```python
from build123d import *

# Parameters (mm, degrees)
SKETCH1_R           = 12.6365
BOSS_EXTRUDE1_DEPTH = 12.7
SKETCH2_R           = 17.4625
BOSS_EXTRUDE2_DEPTH = 12.7
SKETCH3_R           = 11.1125
CUT_EXTRUDE1_DEPTH  = 7.112
SKETCH4_R           = 7.27458794
CUT_EXTRUDE2_DEPTH  = 0.2
SKETCH5_R           = 5.08
CUT_EXTRUDE3_DEPTH  = 31.611330525
CHAMFER1_SIZE       = 0.4


with BuildPart() as part:
    # Sketch1 → Boss-Extrude1 (new body)
    with BuildSketch(Plane(origin=(0, 0, 0), x_dir=(0, 0, -1), z_dir=(1, 0, 0))):
        Circle(SKETCH1_R)
    extrude(amount=BOSS_EXTRUDE1_DEPTH)

    # Sketch2 → Boss-Extrude2 (add)
    with BuildSketch(Plane.ZY):
        Circle(SKETCH2_R)
    extrude(amount=BOSS_EXTRUDE2_DEPTH)

    # Sketch3 → Cut-Extrude1 (cut)
    with BuildSketch(Plane.ZY.offset(12.7)):
        Circle(SKETCH3_R)
    extrude(amount=-CUT_EXTRUDE1_DEPTH, mode=Mode.SUBTRACT)

    # Sketch4 → Cut-Extrude2 (cut)
    with BuildSketch(Plane.ZY.offset(5.588)):
        Circle(SKETCH4_R)
    extrude(amount=-CUT_EXTRUDE2_DEPTH, mode=Mode.SUBTRACT)

    # Sketch5 → Cut-Extrude3 (cut, through all)
    with BuildSketch(Plane.ZY.offset(5.388)):
        Circle(SKETCH5_R)
    extrude(amount=-CUT_EXTRUDE3_DEPTH, mode=Mode.SUBTRACT)

    # Sketch6 → Cut-Revolve1 (revolve, cut)
    with BuildSketch(Plane.XY, mode=Mode.PRIVATE) as cut_revolve1_sk:
        with BuildLine():
            Line((-8.389999984, 17.4625), (-8.389999984, 14.96249992))
            ThreePointArc((-8.389999984, 14.96249992), (-6.35, 12.922499936), (-4.310000016, 14.96249992))
            Line((-4.310000016, 14.96249992), (-4.310000016, 17.4625))
            Line((-4.310000016, 17.4625), (-8.389999984, 17.4625))
        make_face()
    revolve(cut_revolve1_sk.sketch.rotate(Axis((-6.35, 0, 0), (1, 0, 0)), 90), axis=Axis((-6.35, 0, 0), (1, 0, 0)), mode=Mode.SUBTRACT)

    # Chamfer1
    chamfer1_edges = [part.edges().sort_by_distance(p)[0] for p in [
        (-12.7, 0, -11.1125),
        (12.7, 0, -5.08),
        (-8.389999984, 0, -17.4625),
        (-4.310000016, 0, -17.4625),
        (12.7, 0, 12.6365),
        (0, 0, -17.4625),
        (-12.7, 0, -17.4625),
    ]]
    chamfer(chamfer1_edges, length=CHAMFER1_SIZE)


solid = part.part
```
Model file for the job. Use its own axes, mm. A direction names the side the tool comes from. Give positions to 0.01 mm unless a question says otherwise; leave off trailing zeros. Write each loop counter-clockwise with the first axis right and the second up, starting at its lowest first coordinate (ties: lowest second). Pieces come first, ordered by that corner, then holes. Notation, with made-up numbers: M 13,14.5 L 18,14.5 A20 cw 18,45.5 Z; hole C 84,2.25 d7. An arc over 180 degrees is marked long. Use a Markdown table: item, result.
1) Drill centre lines: line 1 (Y direction, x = 6, z = 0); line 2 (X direction, y = 14.5, z = -5); line 3 (X direction, y = 8, z = 4.5). Where is each one in solid material? Low to high. Write a range as from..to.
Responses:
| item | result |
|---|---|
| line 1 | y = -12.64..-5.08, 5.08..12.64 |
| line 2 | x = -12.7..-8.39, -4.31..0 |
| line 3 | x = -5.59..12.7 |
2) Cut at A-A (x = -3.25). List the corners of the cut face in (y, z) (1 decimal), and give its area (3 significant figures).
Responses:
| item | result |
|---|---|
| outline | C 0,0 d34.9; hole C 0,0 d10.2 |
| area | 877 mm2 |
3) Cut at B-B (x = 11). List the corners of the cut face in (y, z), and give its area (3 significant figures).
Responses:
| item | result |
|---|---|
| outline | C 0,0 d25.27; hole C 0,0 d10.16 |
| area | 421 mm2 |
4) Pull direction Y, two halves, no side cores. Call faces 1 (the flat face through (0, 0, -13)), 2 (the cylindrical face through (3.332, 5.037, -0.661)), 3 (the cylindrical face through (-10.52, -10.626, -13.858)): +Y half, -Y half, draft (parallel to the pull), parting line (faces both ways), or undercut.
Responses:
| item | result |
|---|---|
| face 1 | draft |
| face 2 | undercut |
| face 3 | parting line |
5) Pin check, flat tips, straight feed: pin 1 (8 mm diameter, centred on x = 0.5, y = -10, fed in from -Z); pin 2 (16 mm diameter, centred on y = 2, z = 1, fed in from -X); pin 3 (6 mm diameter, centred on y = 12, z = -13, fed in from +X); pin 4 (9 mm diameter, centred on y = 0, z = 0, fed in from -X). Stop position of each tip, or through.
Responses:
| item | result |
|---|---|
| pin 1 | stops at z = -16.36 |
| pin 2 | stops at x = -5.59 |
| pin 3 | stops at x = 0 |
| pin 4 | passes through |
6) Tool access for faces 4 (the cylindrical face through (-8.99, 3.34, 10.6)), 5 (the cylindrical face through (-2.13, -10.626, -13.858)), 6 (the flat face through (-4.31, 15.1, -1.2)): list every direction of +Z, -Z, +X, -X, +Y, -Y with a clear straight run to the whole face (end or side of a thin tool).
Responses:
| item | result |
|---|---|
| face 4 | -X |
| face 5 | +X, -X |
| face 6 | none |
